Input: dimensioned drawing with shaded views. Units: mm. Origin: part minimum x, y, z. A direction names the side the tool comes from. Round coordinates to 2 decimals unless told otherwise and drop trailing zeros. Loops run counter-clockwise (first coordinate to the right, second up) from the corner with the lowest first, then second, coordinate; pieces in that order, holes last.
1) Draft query along X for the marked faces 1, 2 and 3. Return one class per face: pulls with the +X half, pulls with the -X half, needs draft (parallel to the pull), parting line crosses it, or undercut.
2) Ray query, line 1 along X through (y, z) = (0.95, 20); line 2 along Y through (x, z) = (11, 1.5); line 3 along Z through (x, y) = (9, 0.75). Return the intervals inside material, ascending.
3) Section B-B, the plane z = 20. Return loops of the section in (x, y).
4) Section C-C, the plane x = 6.5. Return loops of the section in (y, z), and give its area (3 significant figures).
5) First-contact query: pin 1 (4 mm diameter, centred on x = 18.5, z = 20, fed in from +Y); pin 2 (3 mm diameter, centred on x = 11.5, y = 1.5, fed in from -Z); pin 3 (6.5 mm diameter, centred on x = 12.5, z = 1.5, fed in from -Y); pin 4 (3 mm diameter, centred on x = 2.5, z = 20, fed in from -Y). Flat tips, straight axial feed; report the tip coordinate or a pass-through.
6) Section D-D, the plane y = 1.5. Return loops of the section in (x, z).
7) Section A-A, the plane x = 2.5. Return loops of the section in (y, z), and give its area (3 significant figures).
8) Access query for the marked faces 4, 5 and 6. Directions: +Z, -Z, +X, -X, +Y, -Y. A direction counts if a zero-diameter tool reaches every point of the face in a straight line with its end or side. Return the directions, or none.
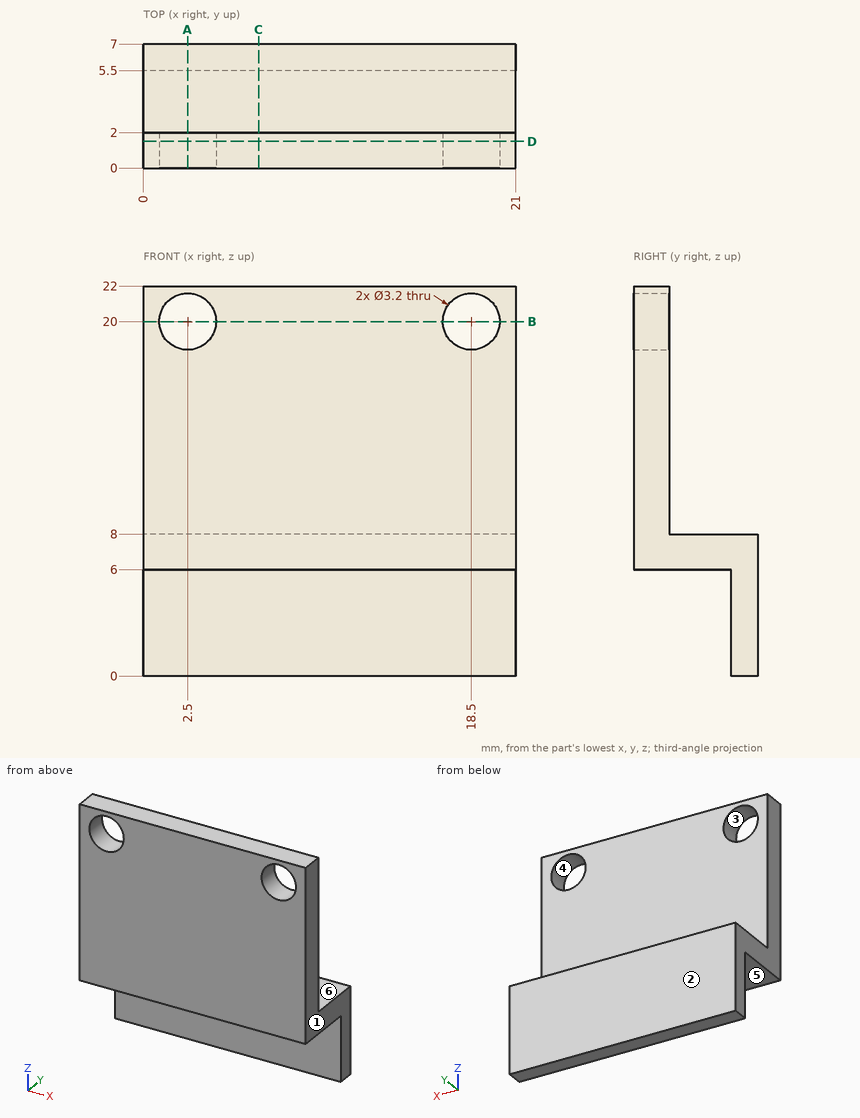
Final values:
1. face 1: pulls with the +X half
1. face 2: needs draft
1. face 3: undercut
2. line 1: x = 0 to 0.9, 4.1 to 16.9, 20.1 to 21
2. line 2: y = 5.5 to 7
2. line 3: z = 6 to 22
3. outline: (0, 0) - (0.9, 0) - (0.9, 2) - (0, 2) - close; (4.1, 0) - (16.9, 0) - (16.9, 2) - (4.1, 2) - close; (20.1, 0) - (21, 0) - (21, 2) - (20.1, 2) - close
4. outline: (0, 6) - (5.5, 6) - (5.5, 0) - (7, 0) - (7, 8) - (2, 8) - (2, 22) - (0, 22) - close
4. area: 51.0 mm2
5. pin 1: stops at y = 2
5. pin 2: stops at z = 6
5. pin 3: stops at y = 5.5
5. pin 4: passes through
6. outline: (0, 6) - (21, 6) - (21, 22) - (0, 22) - close; hole circle Ø3.2 at (2.5, 20); hole circle Ø3.2 at (18.5, 20)
7. outline: (0, 6) - (5.5, 6) - (5.5, 0) - (7, 0) - (7, 8) - (2, 8) - (2, 18.4) - (0, 18.4) - close; (0, 21.6) - (2, 21.6) - (2, 22) - (0, 22) - close
7. area: 44.6 mm2
8. face 4: +Y, -Y
8. face 5: -Z, +X, -X, -Y
8. face 6: +Z, +X, -X, +Y
